Build history of the part. All positions in model axes, mm. Face numbers are marked on the shaded views. Round coordinates to 2 decimals unless told otherwise and drop trailing zeros. Loops run counter-clockwise (first coordinate to the right, second up) from the corner with the lowest first, then second, coordinate; pieces in that order, holes last. Notation, with made-up numbers: (-39.75, 54) -> (-35.75, 54) arc R21 ccw to (-35.75, 89) -> close; hole circle Ø11 at (73, -14.5). An arc over 180 degrees is marked (long way). Put each result on its own line as item: value. Start each with the question number.
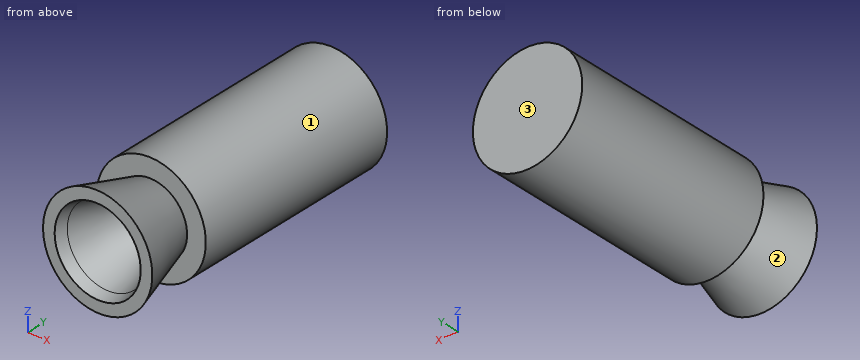
```python
from build123d import *


with BuildPart() as part:
    # Esquisse1 → Révolution1 (revolve)
    with BuildSketch(Plane.XY):
        Polygon((-6.63246603, 74.857346398), (-45.63246603, 74.857346398), (-45.63246603, -98.179299131), (-25.446506602, -98.179299131), (-42.255365298, -155.142653602), (-45.20618497, -165.142653602), (-55.63246603, -165.142653602), (-38.823607333, -108.179299131), (-55.63246603, -108.179299131), (-55.63246603, 84.857346398), (-6.63246603, 84.857346398), align=None)
    revolve(axis=Axis((-6.63246603, 84.857346398, 0), (0, -1, 0)))


solid = part.part
```
Item 1: Cut at C-C on y = -134.5. Write the cut outline in (x, z), then the cut area to 3 significant figures.
Item 2: Pull direction Y, two halves, no side cores. Call the marked faces 1, 2 and 3: +Y half, -Y half, draft (parallel to the pull), parting line (faces both ways), or undercut.
Item 3: Wall check: line 1 (X direction, y = -41, z = 0); line 2 (Z direction, x = -5.5, y = 57.5); line 3 (X direction, y = 23, z = 32.5). Give the ranges that are in metal, low to high. Write a range as from..to.
Item 4: Cut at B-B on z = 33. State how many separate pieces and enclosed holes the cut face has, then the cut area to 3 significant figures.
Item 5: Drop flat-ended pins along their axis: pin 1 (2 mm diameter, centred on x = 22, y = 19.5, fed in from -Z); pin 2 (10 mm diameter, centred on x = -5, y = -126.5, fed in from -Z); pin 3 (1.5 mm diameter, centred on x = -21.5, y = 53.5, fed in from -Z). Give the stop position or say it passes through.
Item 6: Cut at A-A on y = -86.5. Write the cut outline in (x, z), then the cut area to 3 significant figures.
Ans:
1. outline: circle Ø79.92 at (-6.63, 0); hole circle Ø59.06 at (-6.63, 0)
1. area: 2,280 mm2
2. face 1: draft
2. face 2: undercut
2. face 3: +Y half
3. line 1: x = -55.63..-45.63, 32.37..42.37
3. line 2: z = -48.99..-38.98, 38.98..48.99
3. line 3: x = -43.3..-28.19, 14.93..30.04
4. separate pieces: 2
4. enclosed holes: 1
4. area: 8,810 mm2
5. pin 1: stops at z = -40.47
5. pin 2: stops at z = -39.05
5. pin 3: stops at z = -46.92
6. outline: circle Ø98 at (-6.63, 0); hole circle Ø78 at (-6.63, 0)
6. area: 2,760 mm2
